```python
from build123d import *

# Parameters (mm, degrees)
BOSS_EXTRUDE1_DEPTH     = 20
SKETCH2_R               = 18
BOSS_EXTRUDE2_DEPTH     = 65
SKETCH3_R               = 18.5
BOSS_EXTRUDE3_DEPTH     = 308
SKETCH4_R               = 8.75
CUT_EXTRUDE1_DEPTH      = 203.2
SKETCH8_R               = 1
CUT_EXTRUDE2_DEPTH      = 20
SKETCH9_R               = 1.5
BOSS_EXTRUDE4_DEPTH     = 2
CUT_EXTRUDE3_DEPTH      = 1
SKETCH11_R              = 1
BOSS_EXTRUDE5_DEPTH     = 20
MIRROR2_COPY_1_SKETCH_R = 1
MIRROR2_COPY_1_DEPTH    = 20
MIRROR2_COPY_2_SKETCH_R = 1.5
MIRROR2_COPY_2_DEPTH    = 2
MIRROR2_COPY_3_DEPTH    = 1
MIRROR2_COPY_4_SKETCH_R = 1
MIRROR2_COPY_4_DEPTH    = 20
MIRROR2_COPY_5_SKETCH_R = 1
MIRROR2_COPY_5_DEPTH    = 20
MIRROR2_COPY_6_SKETCH_R = 1
MIRROR2_COPY_6_DEPTH    = 20


with BuildPart() as part:
    # Sketch1 → Boss-Extrude1 (new body)
    with BuildSketch(Plane(origin=(0, 0, 0), x_dir=(1, 0, 0), z_dir=(0, 1, 0))):
        with BuildLine():
            Line((30, 22.5), (-30, 22.5))
            ThreePointArc((-30, 22.5), (-52.5, 0), (-30, -22.5))
            Line((-30, -22.5), (30, -22.5))
            ThreePointArc((30, -22.5), (52.5, 0), (30, 22.5))
        make_face()
    extrude(amount=BOSS_EXTRUDE1_DEPTH)

    # Sketch2 → Boss-Extrude2 (add)
    with BuildSketch(Plane(origin=(0, 20, 0), x_dir=(1, 0, 0), z_dir=(0, 1, 0))):
        with Locations(Location((-30, 0, 0), (0, 0, 270))):
            Circle(SKETCH2_R)
    extrude(amount=BOSS_EXTRUDE2_DEPTH)

    # Sketch3 → Boss-Extrude3 (add)
    with BuildSketch(Plane(origin=(0, 20, 0), x_dir=(1, 0, 0), z_dir=(0, 1, 0))):
        with Locations(Location((30, 0, 0), (0, 0, 270))):
            Circle(SKETCH3_R)
    extrude(amount=BOSS_EXTRUDE3_DEPTH)

    # Sketch4 → Cut-Extrude1 (cut)
    with BuildSketch(Plane(origin=(0, 328, 0), x_dir=(1, 0, 0), z_dir=(0, 1, 0))):
        with Locations(Location((30, 0, 0), (0, 0, 270))):
            Circle(SKETCH4_R)
    extrude(amount=-CUT_EXTRUDE1_DEPTH, mode=Mode.SUBTRACT)

    # Sketch8 → Cut-Extrude2 (cut)
    with BuildSketch(Plane(origin=(0, 20, 0), x_dir=(1, 0, 0), z_dir=(0, 1, 0))):
        with Locations(Location((-30, -20.25, 0), (0, 0, 270))):
            Circle(SKETCH8_R)
    cut_extrude2 = extrude(amount=-CUT_EXTRUDE2_DEPTH, mode=Mode.SUBTRACT)

    # Sketch9 → Boss-Extrude4 (add)
    with BuildSketch(Plane(origin=(0, 20, 0), x_dir=(1, 0, 0), z_dir=(0, 1, 0))):
        with Locations(Location((-30, -20.25, 0), (0, 0, 270))):
            Circle(SKETCH9_R)
    boss_extrude4 = extrude(amount=BOSS_EXTRUDE4_DEPTH)

    # Sketch10 → Cut-Extrude3 (cut)
    with BuildSketch(Plane(origin=(0, 22, 0), x_dir=(1, 0, 0), z_dir=(0, 1, 0))):
        Polygon((-29.133974596, -20.75), (-29.133974596, -19.75), (-30, -19.25), (-30.866025404, -19.75), (-30.866025404, -20.75), (-30, -21.25), align=None)
    cut_extrude3 = extrude(amount=-CUT_EXTRUDE3_DEPTH, mode=Mode.SUBTRACT)

    # Sketch11 → Boss-Extrude5 (add)
    with BuildSketch(Plane.XZ.offset(-20)):
        with Locations((-30, 20.25)):
            Circle(SKETCH11_R)
    boss_extrude5 = extrude(amount=BOSS_EXTRUDE5_DEPTH)

    # Mirror1: Cut-Extrude2, Boss-Extrude4, Cut-Extrude3, Boss-Extrude5 across plane
    add(cut_extrude2.mirror(Plane(origin=(0, 0, 0), x_dir=(0, 0, 1), z_dir=(1, 0, 0))), mode=Mode.SUBTRACT)
    add(boss_extrude4.mirror(Plane(origin=(0, 0, 0), x_dir=(0, 0, 1), z_dir=(1, 0, 0))))
    add(cut_extrude3.mirror(Plane(origin=(0, 0, 0), x_dir=(0, 0, 1), z_dir=(1, 0, 0))), mode=Mode.SUBTRACT)
    add(boss_extrude5.mirror(Plane(origin=(0, 0, 0), x_dir=(0, 0, 1), z_dir=(1, 0, 0))))

    # Mirror2: Boss-Extrude4, Cut-Extrude3 across plane
    add(boss_extrude4.mirror(Plane.XY))
    add(cut_extrude3.mirror(Plane.XY), mode=Mode.SUBTRACT)

    # Mirror2 copy 1 sketch → Mirror2 copy 1 (cut)
    with BuildSketch(Plane(origin=(0, 20, 0), x_dir=(-1, 0, 0), z_dir=(0, 1, 0))):
        with Locations(Location((-30, -20.25, 0), (0, 0, 270))):
            Circle(MIRROR2_COPY_1_SKETCH_R)
    extrude(amount=-MIRROR2_COPY_1_DEPTH, mode=Mode.SUBTRACT)

    # Mirror2 copy 2 sketch → Mirror2 copy 2 (add)
    with BuildSketch(Plane(origin=(0, 20, 0), x_dir=(-1, 0, 0), z_dir=(0, 1, 0))):
        with Locations(Location((-30, -20.25, 0), (0, 0, 270))):
            Circle(MIRROR2_COPY_2_SKETCH_R)
    extrude(amount=MIRROR2_COPY_2_DEPTH)

    # Mirror2 copy 3 sketch → Mirror2 copy 3 (cut)
    with BuildSketch(Plane(origin=(0, 22, 0), x_dir=(-1, 0, 0), z_dir=(0, 1, 0))):
        Polygon((-29.133974596, -20.75), (-29.133974596, -19.75), (-30, -19.25), (-30.866025404, -19.75), (-30.866025404, -20.75), (-30, -21.25), align=None)
    extrude(amount=-MIRROR2_COPY_3_DEPTH, mode=Mode.SUBTRACT)

    # Mirror2 copy 4 sketch → Mirror2 copy 4 (add)
    with BuildSketch(Plane(origin=(0, 20, 0), x_dir=(-1, 0, 0), z_dir=(0, -1, 0))):
        with Locations((-30, 20.25)):
            Circle(MIRROR2_COPY_4_SKETCH_R)
    extrude(amount=MIRROR2_COPY_4_DEPTH)

    # Mirror2 copy 5 sketch → Mirror2 copy 5 (cut)
    with BuildSketch(Plane(origin=(0, 20, 0), x_dir=(1, 0, 0), z_dir=(0, 1, 0))):
        with Locations((-30, 20.25)):
            Circle(MIRROR2_COPY_5_SKETCH_R)
    extrude(amount=-MIRROR2_COPY_5_DEPTH, mode=Mode.SUBTRACT)

    # Mirror2 copy 6 sketch → Mirror2 copy 6 (add)
    with BuildSketch(Plane.XZ.offset(-20)):
        with Locations((-30, -20.25)):
            Circle(MIRROR2_COPY_6_SKETCH_R)
    extrude(amount=MIRROR2_COPY_6_DEPTH)


solid = part.part
```
Work out the finished part from the listing and answer in its coordinate system (mm). A direction names the side the tool comes from. Give positions to 0.01 mm unless a question says otherwise; leave off trailing zeros. Order: outer loops, then holes, each group sorted by start corner. A loop starts at its lowest first (then second) coordinate and runs counter-clockwise, first axis right, second up. Notation, with made-up numbers: (-24.75, 74.5) -> (-2.75, 74.5) arc R27 cw to (-2.75, 96.5) -> close; hole circle Ø8 at (55, 45.25). An arc over 180 degrees is marked (long way). Answer as CSV lines item,"result". Start each with the question number.
(1) Which of the six approach directions +Z, -Z, +X, -X, +Y, -Y give full straight-line access (tool end or side, diameter ignored) to faces 4 (the flat face through (0, 10, 22.5)), 5 (the flat face through (-30, 85, 0)), 6 (the cylindrical face through (11.94, 171.84, -4.01))?
(2) Section B-B, the plane y = 61 is taken. Write down the section's boundary in (x, z).
(3) Each of these flat-tipped pins is pushed along its axis until it touches: pin 1 Ø10.5 at (x, z) = (30, 0) entering from -Y; pin 2 Ø0.8 at (y, z) = (21.5, -20.5) entering from -X; pin 3 Ø3 at (y, z) = (48.5, 0) entering from +X; pin 4 Ø1.4 at (x, z) = (30, -20.5) entering from +Y. Where does it stop, or does it pass through?
(4) Section A-A, the plane z = 0 is taken. Write down the section's boundary in (x, y), plus the area to 3 significant figures.
(5) Section C-C, the plane x = 16.5 is taken. Write down the section's boundary in (y, z).
(6) For a pull along X with two mould halves and no side action, classify faces 1 (the flat face through (26, 328, 8)), 2 (the flat face through (-1, 20, 0)), 3 (the cylindrical face through (-52.495, 9.86, -0.495)) as released by +X, released by -X, zero draft, split by the parting line, or undercut.
(7) Consider line 1 along X through (y, z) = (217, 0); line 2 along Y through (x, z) = (-43, 7); line 3 along X through (y, z) = (232.5, -7). Determine where each line is inside the solid, lowest interval first.
(8) Section D-D, the plane y = 157 is taken. Write down the section's boundary in (x, z), plus the area to 3 significant figures.
Entries:
1,face 4,"+Z, +X, -X, +Y, -Y"
1,face 5,"+Z, -Z, -X, +Y"
1,face 6,"+Y"
2,outline,"circle Ø36 at (-30, 0); circle Ø37 at (30, 0)"
3,pin 1,"y = 0"
3,pin 2,"x = -31.5"
3,pin 3,"x = 48.5"
3,pin 4,"y = 22"
4,outline,"(-52.5, 0) -> (52.5, 0) -> (52.5, 20) -> (48.5, 20) -> (48.5, 328) -> (38.75, 328) -> (38.75, 124.8) -> (21.25, 124.8) -> (21.25, 328) -> (11.5, 328) -> (11.5, 20) -> (-12, 20) -> (-12, 85) -> (-48, 85) -> (-48, 20) -> (-52.5, 20) -> close"
4,area,"12,300 mm²"
5,outline,"(0, -22.5) -> (20, -22.5) -> (20, -12.65) -> (328, -12.65) -> (328, 12.65) -> (20, 12.65) -> (20, 22.5) -> (0, 22.5) -> close"
6,face 1,"zero draft"
6,face 2,"undercut"
6,face 3,"released by -X"
7,line 1,"11.5 to 21.25, 38.75 to 48.5"
7,line 2,"0 to 85"
7,line 3,"12.88 to 24.75, 35.25 to 47.12"
8,outline,"circle Ø37 at (30, 0); hole circle Ø17.5 at (30, 0)"
8,area,"835 mm²"
